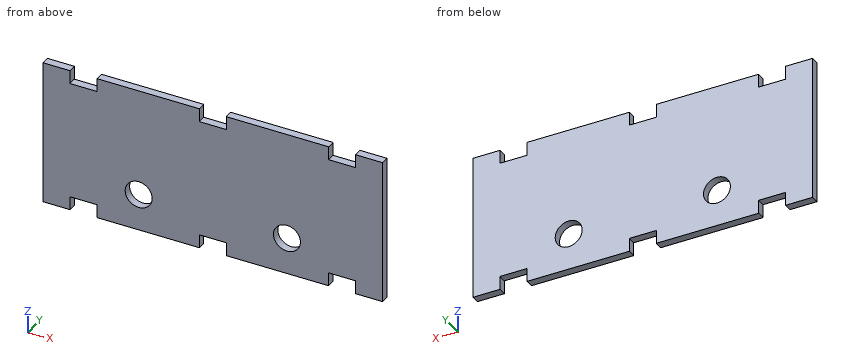
```python
from build123d import *

# Parameters (mm, degrees)
F0_R     = 6.35
F1_DEPTH = 3.81


# Not quite as in the source:
# - a feature names something its author has since deleted; it is built from what else it names


with BuildPart() as f1:
    # F0 (on Front) → F1 (new body)
    with BuildSketch(Plane.XZ):
        Polygon((-80, 34.29), (-80, -34.29), (-67.3, -34.29), (-67.3, -27.94), (-54.6, -27.94), (-54.6, -34.29), (-6.35, -34.29), (-6.35, -27.94), (6.35, -27.94), (6.35, -34.29), (54.6, -34.29), (54.6, -27.94), (67.3, -27.94), (67.3, -34.29), (80, -34.29), (80, 34.29), (67.3, 34.29), (67.3, 27.94), (54.6, 27.94), (54.6, 34.29), (6.35, 34.29), (6.35, 27.94), (-6.35, 27.94), (-6.35, 34.29), (-54.6, 34.29), (-54.6, 27.94), (-67.3, 27.94), (-67.3, 34.29), align=None)
        with Locations((-34.925, -16.8712735176)):
            Circle(F0_R, mode=Mode.SUBTRACT)
        with Locations((34.925, -16.8712735176)):
            Circle(F0_R, mode=Mode.SUBTRACT)
    extrude(amount=F1_DEPTH)


solid = f1.part
```
The listing builds one solid part. Answer for the finished solid, in the listing's coordinates (mm). Give positions to 0.01 mm unless a question says otherwise; leave off trailing zeros. Write each loop counter-clockwise with the first axis right and the second up, starting at its lowest first coordinate (ties: lowest second). Pieces come first, ordered by that corner, then holes. Notation, with made-up numbers: M 29,16 L 50,16 A26 cw 50,53 Z; hole C 25.5,17.5 d2. An arc over 180 degrees is marked long. Write each question's results on one line, items separated by ' | '.
Q1. Consider L1, parallel to X at y = -2.8, z = -16.5; L2, parallel to X at y = -0.6, z = -30; L3, parallel to X at y = -2.35, z = -15. Determine where each line is inside the solid, lowest interval first. Write a range as from..to.
Output values:
L1: -80..-41.26, -28.59..28.59, 41.26..80 | L2: -80..-67.3, -54.6..-6.35, 6.35..54.6, 67.3..80 | L3: -80..-40.99, -28.86..28.86, 40.99..80
Q2. Section D-D, the plane x = -30 is taken. Write down the section's boundary in (y, z), then the cut area to 3 significant figures.
Output values:
outline: M -3.81,-34.29 L 0,-34.29 L 0,-20.88 L -3.81,-20.88 Z; M -3.81,-12.86 L 0,-12.86 L 0,34.29 L -3.81,34.29 Z | area: 231 mm2
Q3. Section C-C, the plane y = -0.8 is taken. Count the separate pieces of the cut face and the enclosed holes in it, then the cut area to 3 significant figures.
Output values:
separate pieces: 1 | enclosed holes: 2 | area: 10,200 mm2
Q4. Section A-A, the plane z = -20 is taken. Write down the section's boundary in (x, y).
Output values:
outline: M -80,-3.81 L -40.45,-3.81 L -40.45,0 L -80,0 Z; M -29.4,-3.81 L 29.4,-3.81 L 29.4,0 L -29.4,0 Z; M 40.45,-3.81 L 80,-3.81 L 80,0 L 40.45,0 Z
Q5. Flat-ended cylindrical pins translate along their axes: P1, Ø1.9, axis at x = 63.5, y = -2, coming from the +Z side; P2, Ø1.9, axis at x = -2.5, y = -2, coming from the -Z side. Find the tip coordinate at first contact, or state that the pin passes through.
Output values:
P1: z = 27.94 | P2: z = -27.94
Q6. Section B-B, the plane x = 32.5 is taken. Write down the section's boundary in (y, z), then the cut area to 3 significant figures.
Output values:
outline: M -3.81,-34.29 L 0,-34.29 L 0,-22.74 L -3.81,-22.74 Z; M -3.81,-11 L 0,-11 L 0,34.29 L -3.81,34.29 Z | area: 217 mm2
